The model under review builds one solid part; all positions refer to its coordinate system, in mm. Face numbers are marked on the shaded views. A direction names the side the tool comes from. Coordinates: 2 decimals unless noted, no trailing zeros. Order: outer loops, then holes, each group sorted by start corner. A loop starts at its lowest first (then second) coordinate and runs counter-clockwise, first axis right, second up. Notation, with made-up numbers: M 26,52.25 L 77,52.25 A12 cw 77,74.25 Z; hole C -12.5,56.5 d9. An arc over 180 degrees is marked long. Write each question's results on one line, items separated by ' | '.
from build123d import *

# Parameters (mm, degrees)
F1_DEPTH  = 12.7
F6_R      = 2.6
F7_DEPTH  = 1.2
F4_R      = 2.6
F8_DEPTH  = 1.2
F5_R      = 2.6
F9_DEPTH  = 1.2
F3_R      = 2.6
F10_DEPTH = 1.2
F2_R      = 2.6
F11_DEPTH = 1.2


with BuildPart() as f1:
    # F0 (on Right) → F1 (new body, symmetric)
    with BuildSketch(Plane.YZ):
        Polygon((7.3323484187, -12.7), (7.3323484187, 12.7), (-14.6646968374, 0), align=None)
    extrude(amount=F1_DEPTH, both=True)

    # F6 (on face) → F7 (cut)
    with BuildSketch(Plane.YZ.offset(12.7)):
        Circle(F6_R)
    extrude(amount=-F7_DEPTH, mode=Mode.SUBTRACT)

    # F4 (on face) → F8 (cut)
    with BuildSketch(Plane(origin=(0, -3.6661742094, -6.35), x_dir=(1, 0, 0), z_dir=(0, -0.5, -0.8660254038))):
        Circle(F4_R)
    extrude(amount=-F8_DEPTH, mode=Mode.SUBTRACT)

    # F5 (on face) → F9 (cut)
    with BuildSketch(Plane(origin=(-12.7, 0, 0), x_dir=(0, -1, 0), z_dir=(-1, 0, 0))):
        Circle(F5_R)
    extrude(amount=-F9_DEPTH, mode=Mode.SUBTRACT)

    # F3 (on face) → F10 (cut)
    with BuildSketch(Plane(origin=(0, 7.3323484187, 0), x_dir=(-1, 0, 0), z_dir=(0, 1, 0))):
        Circle(F3_R)
    extrude(amount=-F10_DEPTH, mode=Mode.SUBTRACT)

    # F2 (on face) → F11 (cut)
    with BuildSketch(Plane(origin=(0, -3.6661742094, 6.35), x_dir=(1, 0, 0), z_dir=(0, -0.5, 0.8660254038))):
        Circle(F2_R)
    extrude(amount=-F11_DEPTH, mode=Mode.SUBTRACT)


solid = f1.part
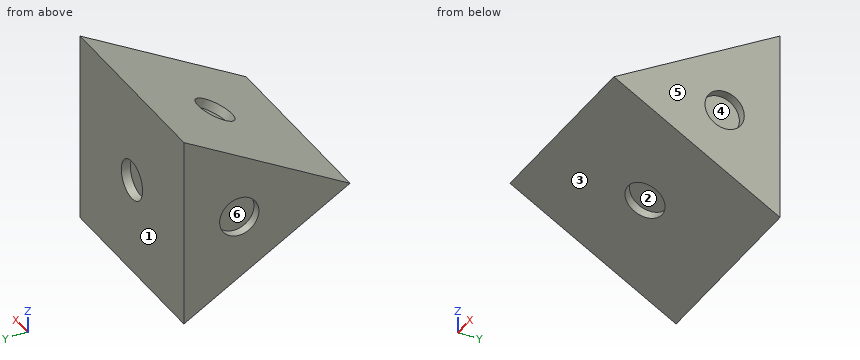
1) For pin 1 (1 mm diameter, centred on x = -3, y = -11.5, fed in from +Z); pin 2 (2.5 mm diameter, centred on y = -1, z = 0.5, fed in from -X); pin 3 (1.6 mm diameter, centred on y = -0.5, z = 1, fed in from +X), all flat-tipped, find the tip position at first contact; note any pin that passes through.
Solutions:
pin 1: z = 2.12 | pin 2: x = -11.5 | pin 3: x = 11.5
2) To check wall thickness, follow line 1 along Z through (x, y) = (12.1, 0); line 2 along Z through (x, y) = (0, 6.9); line 3 along Y through (x, z) = (-1.75, 4.5). State the ranges of each line that lie inside material, in increasing order.
Solutions:
line 1: -8.47 to -2.6, 2.6 to 8.47 | line 2: -12.45 to -2.6, 2.6 to 12.45 | line 3: -6.87 to -4.82, -4.47 to 7.33
3) For the marked faces 4, 5 and 6, list the 3-axis set-ups (+Z, -Z, +X, -X, +Y, -Y) from which the entire face can be reached by the end or side of a thin tool; tool diameter is ignored.
Solutions:
face 4: +X | face 5: +Z, -Z, +X, +Y, -Y | face 6: -X
4) Take a section at B-B on x = -6. State the section outline as (y, z) points.
Solutions:
outline: M -14.66,0 L 7.33,-12.7 L 7.33,12.7 Z
5) Take a section at C-C on z = 1. State the section outline as (x, y) points, plus the area to 3 significant figures.
Solutions:
outline: M -12.7,-12.93 L 12.7,-12.93 L 12.7,-2.4 L 11.5,-2.4 L 11.5,2.4 L 12.7,2.4 L 12.7,7.33 L 2.4,7.33 L 2.4,6.13 L -2.4,6.13 L -2.4,7.33 L -12.7,7.33 L -12.7,2.4 L -11.5,2.4 L -11.5,-2.4 L -12.7,-2.4 Z | area: 497 mm2
6) The part is to be moulded in two halves that separate along Y. For the marked faces 1, 2 and 3, say which applies: pulls with the +Y half, pulls with the -Y half, needs draft (parallel to the pull), parting line crosses it, or undercut.
Solutions:
face 1: pulls with the +Y half | face 2: undercut | face 3: pulls with the -Y half
7) Take a section at D-D on x = 0. State the section outline as (y, z) points.
Solutions:
outline: M -14.66,0 L -5.92,-5.05 L -5.32,-4.01 L -0.81,-6.61 L -1.41,-7.65 L 7.33,-12.7 L 7.33,-2.6 L 6.13,-2.6 L 6.13,2.6 L 7.33,2.6 L 7.33,12.7 L -1.41,7.65 L -0.81,6.61 L -5.32,4.01 L -5.92,5.05 Z
8) Take a section at A-A on y = 0. State the section outline as (x, z) points, plus the area to 3 significant figures.
Solutions:
outline: M -12.7,-8.47 L 12.7,-8.47 L 12.7,-2.6 L 11.5,-2.6 L 11.5,2.6 L 12.7,2.6 L 12.7,8.47 L -12.7,8.47 L -12.7,2.6 L -11.5,2.6 L -11.5,-2.6 L -12.7,-2.6 Z | area: 418 mm2
